Check sheet for the modelled part. Datum: model origin and axes. Units: mm. A direction names the side the tool comes from. Round coordinates to 2 decimals unless told otherwise and drop trailing zeros. Order: outer loops, then holes, each group sorted by start corner. A loop starts at its lowest first (then second) coordinate and runs counter-clockwise, first axis right, second up. Notation, with made-up numbers: (-33, -20.5) -> (12, -20.5) arc R21 cw to (12, -16.5) -> close; hole circle Ø3 at (59, 4.25). An arc over 180 degrees is marked (long way). Answer in a Markdown table with one row per item. Add a question column.
1. Depth check by flat-ended pin: P1, Ø6, axis at x = -12.05, y = 52.61, coming from the +Z side; P2, Ø7, axis at x = -12.05, y = 52.61, coming from the -Z side; P3, Ø3, axis at x = -12.05, y = -55.85, coming from the +Z side. Enter the tip coordinate at first touch or a pass-through.
2. Sectioned sample at B-B, the plane x = -17.5. Record the boundary of the cut face in (y, z).
3. Material ranges on L1, parallel to X at y = -55.85, z = -1.35; L2, parallel to X at y = -55.85, z = -0.25; L3, parallel to Y at x = 5, z = -0.55, recorded low to high. Write a range as from..to.
4. Access from +Z, -Z, +X, -X, +Y, -Y to the whole of each face (thin tool, end or side, straight path). Record for faces 5 (the flat face through (-2, -56, -2)), 6 (the flat face through (-10, -54, -1)), 7 (the cylindrical face through (7.195, -58.235, -1.507)).
5. Draft check along Y on faces 1 (the flat face through (-2, 46.45, -3)), 2 (the cylindrical face through (-12.23, 56.61, -0.51)), 3 (the flat face through (11, 53, -1)), 4 (the flat face through (-2, 1, 0)). Enter one of: +Y half, -Y half, draft (parallel to the pull), parting line (faces both ways), or undercut.
6. Sectioned sample at A-A, the plane y = -55.85. Record the boundary of the cut face in (x, z), then the cut area to 3 significant figures.
Autodesk Inventor part; units mm, degrees
ref_plane "YZ Plane" through (0, 0, 0) normal (1, 0, 0) x (0, 1, 0)
ref_plane "XZ Plane" through (0, 0, 0) normal (0, 1, 0) x (-1, 0, 0)
ref_plane "XY Plane" through (0, 0, 0) normal (0, 0, 1) x (1, 0, 0)
sketch "Sketch1" plane through (0, 0, 0) normal (0, 0, 1) x (1, 0, 0)
  line L0 (-22.0545, -63.25) -> (17.9455, -63.25)
  line L1 (17.9455, -63.25) -> (17.9455, 63.25)
  line L2 (17.9455, 63.25) -> (-22.0545, 63.25)
  line L3 (-22.0545, 63.25) -> (-22.0545, -63.25)
  line L4 (-22.0545, -63.25) -> (17.9455, 63.25) construction
  line L5 (17.9455, -63.25) -> (-22.0545, 63.25) construction
  line L6 (-22.0545, -63.25) -> (17.9455, -63.25)
  line L7 (17.9455, -63.25) -> (17.9455, -48.45)
  line L8 (17.9455, -48.45) -> (-22.0545, -48.45)
  line L9 (-22.0545, -48.45) -> (-22.0545, -63.25)
  line L10 (-22.0545, -55.85) -> (17.9455, -55.85) construction
  line L11 (-2.0545, -55.85) -> (7.9455, -55.85) construction
  line L12 (-2.0545, -55.85) -> (-12.0545, -55.85) construction
  line L13 (-22.0545, 63.25) -> (17.9455, 63.25)
  line L14 (17.9455, 63.25) -> (17.9455, 46.45)
  line L15 (17.9455, 46.45) -> (-22.0545, 46.45)
  line L16 (-22.0545, 46.45) -> (-22.0545, 63.25)
  line L17 (-22.0545, 46.45) -> (-22.0545, 52.614) construction
  line L18 (-22.0545, 52.614) -> (17.9455, 52.614) construction
  line L19 (-2.0545, 52.614) -> (7.9455, 52.614) construction
  line L20 (-2.0545, 52.614) -> (-12.0545, 52.614) construction
  line L21 (-22.0545, 46.45) -> (17.9455, 46.45)
  line L22 (17.9455, 46.45) -> (17.9455, -48.45)
  line L23 (17.9455, -48.45) -> (-22.0545, -48.45)
  line L24 (-22.0545, -48.45) -> (-22.0545, 46.45)
  point P0 (0, 0)
  point P1 (-2.0545, 0)
  dimension "d0" = 40
  dimension "d1" = 126.5
  dimension "d4" = 14.8
  dimension "d5" = 10
  dimension "d6" = 10
  dimension "d9" = 16.8
  dimension "d10" = 6.164
  dimension "d11" = 10
  dimension "d12" = 10
extrude "Extrusion1" add sketch "Sketch1" against normal blind 2
extrude "Extrusion2" add sketch "Sketch1" against normal blind 4 contours L3 L15 L1 L8
hole "Hole1" at (-12.0545, 52.614, 0) at (7.9455, 52.614, 0) at (-12.0545, -55.85, 0) at (7.9455, -55.85, 0) direction (0, 0, -1) diameter 5 end through all counterbore diameter 8 counterbore depth 1
properties part number "BatteryCover"
Answer key:
| question | item | result |
|---|---|---|
| 1 | P1 | stops at z = -1 |
| 1 | P2 | stops at z = -2 |
| 1 | P3 | passes through |
| 2 | outline | (-63.25, -2) -> (-48.45, -2) -> (-48.45, -4) -> (46.45, -4) -> (46.45, -2) -> (63.25, -2) -> (63.25, 0) -> (-63.25, 0) -> close |
| 3 | L1 | x = -22.05..-14.55, -9.55..5.45, 10.45..17.95 |
| 3 | L2 | x = -22.05..-16.05, -8.05..3.95, 11.95..17.95 |
| 3 | L3 | y = -63.25..-58.56, -53.14..49.91, 55.32..63.25 |
| 4 | face 5 | -Z, +X, -X, -Y |
| 4 | face 6 | +Z |
| 4 | face 7 | +Z, -Z |
| 5 | face 1 | +Y half |
| 5 | face 2 | undercut |
| 5 | face 3 | undercut |
| 5 | face 4 | draft |
| 6 | outline | (-22.05, -2) -> (-14.55, -2) -> (-14.55, -1) -> (-16.05, -1) -> (-16.05, 0) -> (-22.05, 0) -> close; (-9.55, -2) -> (5.45, -2) -> (5.45, -1) -> (3.95, -1) -> (3.95, 0) -> (-8.05, 0) -> (-8.05, -1) -> (-9.55, -1) -> close; (10.45, -2) -> (17.95, -2) -> (17.95, 0) -> (11.95, 0) -> (11.95, -1) -> (10.45, -1) -> close |
| 6 | area | 54.0 mm² |
